Input: part model. Units: mm. Frame: model coordinates. A direction names the side the tool comes from. Coordinates: 2 decimals unless noted, no trailing zeros. Order: outer loops, then holes, each group sorted by start corner. A loop starts at its lowest first (then second) coordinate and runs counter-clockwise, first axis right, second up.
from build123d import *

# Parameters (mm, degrees)
SKETCH1_W                = 131
SKETCH1_H                = 50
BOSS_EXTRUDE6_DEPTH      = 5
SKETCH11_W               = 33
SKETCH11_H               = 40
CUT_EXTRUDE7_DEPTH       = 5
BOSS_EXTRUDE7_DEPTH      = 30
SKETCH13_W               = 30
SKETCH13_H               = 25
CUT_EXTRUDE8_DEPTH       = 66.5
CUT_EXTRUDE8_DEPTH_BACK  = 66.5
SKETCH15_R               = 1.85
CUT_EXTRUDE10_DEPTH      = 26
CUT_EXTRUDE10_DEPTH_BACK = 26


with BuildPart() as part:
    # Sketch1 → Boss-Extrude6 (new body)
    with BuildSketch(Plane(origin=(0, 0, 0), x_dir=(1, 0, 0), z_dir=(0, 1, 0))):
        Rectangle(SKETCH1_W, SKETCH1_H)
    extrude(amount=BOSS_EXTRUDE6_DEPTH)

    # Sketch11 → Cut-Extrude7 (cut)
    with BuildSketch(Plane(origin=(0, 0, 0), x_dir=(1, 0, 0), z_dir=(0, 1, 0))):
        with Locations((38, 0)):
            Rectangle(SKETCH11_W, SKETCH11_H)
        Rectangle(SKETCH11_W, SKETCH11_H)
        with Locations((-38, 0)):
            Rectangle(SKETCH11_W, SKETCH11_H)
    extrude(amount=CUT_EXTRUDE7_DEPTH, mode=Mode.SUBTRACT)

    # Sketch12 → Boss-Extrude7 (add)
    with BuildSketch(Plane(origin=(0, 0, 0), x_dir=(1, 0, 0), z_dir=(0, 1, 0))):
        Polygon((-65.5, -20), (-65.5, -25), (-59, -25), (-16.5, -25), (-16.5, -20), (-60.5, -20), (-60.5, 20), (-16.5, 20), (-16.5, 25), (-59, 25), (-65.5, 25), (-65.5, 20), align=None)
        Polygon((49.5, 25), (49.5, 20), (60.5, 20), (60.5, -20), (49.5, -20), (49.5, -25), (65.5, -25), (65.5, 25), align=None)
    extrude(amount=BOSS_EXTRUDE7_DEPTH)

    # Sketch13 → Cut-Extrude8 (cut, two sides)
    with BuildSketch(Plane(origin=(0, 0, 0), x_dir=(0, 0, -1), z_dir=(1, 0, 0))) as cut_extrude8_sk:
        with Locations((0, 17.5)):
            Rectangle(SKETCH13_W, SKETCH13_H)
    extrude(amount=CUT_EXTRUDE8_DEPTH, mode=Mode.SUBTRACT)
    extrude(cut_extrude8_sk.sketch, amount=-CUT_EXTRUDE8_DEPTH_BACK, mode=Mode.SUBTRACT)

    # Sketch15 → Cut-Extrude10 (cut, two sides)
    with BuildSketch(Plane.XY) as cut_extrude10_sk:
        with Locations((-35, 10)):
            Circle(SKETCH15_R)
        with Locations((-35, 20)):
            Circle(SKETCH15_R)
        with Locations((-25, 20)):
            Circle(SKETCH15_R)
        with Locations((-25, 10)):
            Circle(SKETCH15_R)
        with Locations((-45, 20)):
            Circle(SKETCH15_R)
        with Locations((-45, 10)):
            Circle(SKETCH15_R)
    extrude(amount=CUT_EXTRUDE10_DEPTH, mode=Mode.SUBTRACT)
    extrude(cut_extrude10_sk.sketch, amount=-CUT_EXTRUDE10_DEPTH_BACK, mode=Mode.SUBTRACT)


solid = part.part
Item 1: Access query for faces 4 (the face through (-63, 17, 15)), 5 (the face through (-54.5, 2, 0)), 6 (the face through (-39, 15, -20)). Directions: +Z, -Z, +X, -X, +Y, -Y. A direction counts if a zero-diameter tool reaches every point of the face in a straight line with its end or side. Return the directions, or none.
Response values:
face 4: +X, -X, +Y
face 5: +Y, -Y
face 6: +Y
Item 2: Pin query (flat end, axial travel): pin 1 Ø3.5 at (x, y) = (-35, 20) entering from -Z. Return the tip coordinate at first contact, or that it passes through.
Response values:
pin 1: passes through
Item 3: Cut plane A-A on z = 1.5. Return loops of the section in (x, y), then the cut area to 3 significant figures.
Response values:
outline: (-65.5, 0) - (-54.5, 0) - (-54.5, 5) - (-65.5, 5) - close; (-21.5, 0) - (-16.5, 0) - (-16.5, 5) - (-21.5, 5) - close; (16.5, 0) - (21.5, 0) - (21.5, 5) - (16.5, 5) - close; (54.5, 0) - (65.5, 0) - (65.5, 5) - (54.5, 5) - close
area: 160 mm2
Item 4: Cut plane B-B on x = -7. Return loops of the section in (y, z).
Response values:
outline: (0, -25) - (5, -25) - (5, -20) - (0, -20) - close; (0, 20) - (5, 20) - (5, 25) - (0, 25) - close
Item 5: Ray query, probe 1 along Y at (x, z) = (-35, -23.1); probe 2 along X at (y, z) = (2.75, -8); probe 3 along Z at (x, y) = (-23, 14.25). Return the intervals inside material, ascending.
Response values:
probe 1: y = 0 to 8.15, 11.85 to 18.15, 21.85 to 30
probe 2: x = -65.5 to -54.5, -21.5 to -16.5, 16.5 to 21.5, 54.5 to 65.5
probe 3: z = -25 to -20, 20 to 25
Item 6: Cut plane C-C on y = 27.25. Return loops of the section in (x, z), then the cut area to 3 significant figures.
Response values:
outline: (-65.5, -25) - (-16.5, -25) - (-16.5, -20) - (-60.5, -20) - (-60.5, -15) - (-65.5, -15) - close; (-65.5, 15) - (-60.5, 15) - (-60.5, 20) - (-16.5, 20) - (-16.5, 25) - (-65.5, 25) - close; (49.5, -25) - (65.5, -25) - (65.5, -15) - (60.5, -15) - (60.5, -20) - (49.5, -20) - close; (49.5, 20) - (60.5, 20) - (60.5, 15) - (65.5, 15) - (65.5, 25) - (49.5, 25) - close
area: 750 mm2
Item 7: Cut plane D-D on x = -25. Return loops of the section in (y, z), then the cut area to 3 significant figures.
Response values:
outline: (0, -25) - (8.15, -25) - (8.15, -20) - (0, -20) - close; (0, 20) - (8.15, 20) - (8.15, 25) - (0, 25) - close; (11.85, -25) - (18.15, -25) - (18.15, -20) - (11.85, -20) - close; (11.85, 20) - (18.15, 20) - (18.15, 25) - (11.85, 25) - close; (21.85, -25) - (30, -25) - (30, -20) - (21.85, -20) - close; (21.85, 20) - (30, 20) - (30, 25) - (21.85, 25) - close
area: 226 mm2
Item 8: Draft query along X for faces 1 (the face through (-41, 30, 22)), 2 (the face through (0, 2, 20)), 3 (the face through (-39, 15, 20)). Return one class per face: pulls with the +X half, pulls with the -X half, needs draft (parallel to the pull), parting line crosses it, or undercut.
Response values:
face 1: needs draft
face 2: undercut
face 3: undercut
